Verification items for the finished model (mm, model axes). Give positions to 0.01 mm unless a question says otherwise; leave off trailing zeros. Write each loop counter-clockwise with the first axis right and the second up, starting at its lowest first coordinate (ties: lowest second). Pieces come first, ordered by that corner, then holes. Notation, with made-up numbers: (-18.5, 40.25) -> (35.5, 40.25) arc R24 ccw to (35.5, 75.25) -> close; hole circle Ø3 at (-9, 17.5). An arc over 180 degrees is marked (long way). Use CSV: the item, a comma, the result in double quotes. Start each with the question number.
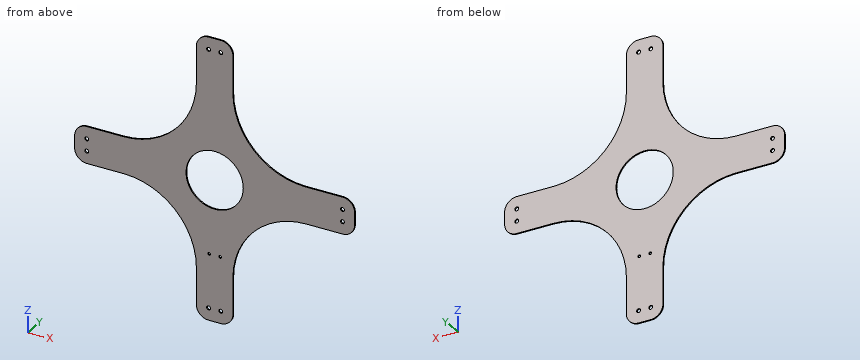
```python
from build123d import *

# Parameters (mm, degrees)
BOSS_EXTRUDE1_DEPTH      = 0.5
M3_CLEARANCE_HOLE1_D     = 3.2
M3_CLEARANCE_HOLE1_DEPTH = 1
SKETCH5_R                = 23.5
CUT_EXTRUDE1_DEPTH       = 1
CUT_EXTRUDE1_DEPTH_BACK  = 2
M2_CLEARANCE_HOLE1_D     = 2.2
M2_CLEARANCE_HOLE1_DEPTH = 1


with BuildPart() as part:
    # Sketch1 → Boss-Extrude1 (new body, symmetric)
    with BuildSketch(Plane(origin=(0, 0, 0), x_dir=(1, 0, 0), z_dir=(0, 1, 0))):
        with BuildLine():
            Line((75, 15), (105, 15))
            ThreePointArc((105, 15), (112.071067812, 12.071067812), (115, 5))
            Line((115, 5), (115, -5))
            ThreePointArc((115, -5), (112.071067812, -12.071067812), (105, -15))
            Line((105, -15), (75, -15))
            ThreePointArc((75, -15), (32.573593129, -32.573593129), (15, -75))
            Line((15, -75), (15, -105))
            ThreePointArc((15, -105), (12.071067812, -112.071067812), (5, -115))
            Line((5, -115), (-5, -115))
            ThreePointArc((-5, -115), (-12.071067812, -112.071067812), (-15, -105))
            Line((-15, -105), (-15, -75))
            ThreePointArc((-15, -75), (-32.573593129, -32.573593129), (-75, -15))
            Line((-75, -15), (-105, -15))
            ThreePointArc((-105, -15), (-112.071067812, -12.071067812), (-115, -5))
            Line((-115, -5), (-115, 5))
            ThreePointArc((-115, 5), (-112.071067812, 12.071067812), (-105, 15))
            Line((-105, 15), (-75, 15))
            ThreePointArc((-75, 15), (-32.573593129, 32.573593129), (-15, 75))
            Line((-15, 75), (-15, 105))
            ThreePointArc((-15, 105), (-12.071067812, 112.071067812), (-5, 115))
            Line((-5, 115), (5, 115))
            ThreePointArc((5, 115), (12.071067812, 112.071067812), (15, 105))
            Line((15, 105), (15, 75))
            ThreePointArc((15, 75), (32.573593129, 32.573593129), (75, 15))
        make_face()
    extrude(amount=BOSS_EXTRUDE1_DEPTH, both=True)

    # M3 Clearance Hole1
    with Locations(Plane(origin=(0, 0.5, 0), x_dir=(1, 0, 0), z_dir=(0, 1, 0))):
        with Locations((-105, 5), (-105, -5), (-5, 105), (5, 105), (105, 5), (105, -5), (5, -105), (-5, -105)):
            Hole(M3_CLEARANCE_HOLE1_D / 2, depth=M3_CLEARANCE_HOLE1_DEPTH)

    # Sketch5 → Cut-Extrude1 (cut, two sides)
    with BuildSketch(Plane(origin=(0, 0.5, 0), x_dir=(1, 0, 0), z_dir=(0, 1, 0))) as cut_extrude1_sk:
        Circle(SKETCH5_R)
    extrude(amount=CUT_EXTRUDE1_DEPTH, mode=Mode.SUBTRACT)
    extrude(cut_extrude1_sk.sketch, amount=-CUT_EXTRUDE1_DEPTH_BACK, mode=Mode.SUBTRACT)

    # M2 Clearance Hole1
    with Locations(Plane(origin=(0, 0.5, 0), x_dir=(1, 0, 0), z_dir=(0, 1, 0))):
        with Locations((-4.5, 61), (4.5, 61)):
            Hole(M2_CLEARANCE_HOLE1_D / 2, depth=M2_CLEARANCE_HOLE1_DEPTH)


solid = part.part
```
(1) Go/stop test with flat-tipped pins: pin 1 (0.5 mm diameter, centred on x = -89, y = 0, fed in from +Z); pin 2 (5 mm diameter, centred on x = -5, z = -105, fed in from +Y); pin 3 (0.5 mm diameter, centred on y = 0, z = -88.5, fed in from +X). Record where each tip stops, or that it passes through.
(2) Section check B-B on x = 79. Record the cut outline in (y, z).
(3) Thickness scan on line 1 (Z direction, x = 105, y = -0.15); line 2 (Z direction, x = -5, y = 0.1). Record the ranges inside material, lowest first. Write a range as from..to.
(4) Section check C-C on z = -98. Record the cut outline in (x, y).
(5) Section check A-A on y = -0.1. Give the number of separate pieces and of enclosed holes in the cut face, then the cut area to 3 significant figures.
Data:
1,pin 1,"stops at z = 15"
1,pin 2,"stops at y = 0.5"
1,pin 3,"stops at x = 15"
2,outline,"(-0.5, -15) -> (0.5, -15) -> (0.5, 15) -> (-0.5, 15) -> close"
3,line 1,"z = -15..-6.6, -3.4..3.4, 6.6..15"
3,line 2,"z = -115..-106.6, -103.4..-61.98, -60.02..-22.96, 22.96..103.4, 106.6..115"
4,outline,"(-15, -0.5) -> (15, -0.5) -> (15, 0.5) -> (-15, 0.5) -> close"
5,separate pieces,"1"
5,enclosed holes,"11"
5,area,"14,000 mm2"
